For this review, take the finished solid that the model builds, in its own axes (mm). A direction names the side the tool comes from. Give positions to 0.01 mm unless a question says otherwise; leave off trailing zeros. Order: outer loops, then holes, each group sorted by start corner. A loop starts at its lowest first (then second) coordinate and runs counter-clockwise, first axis right, second up.
Autodesk Inventor part; units mm, degrees
ref_plane "YZ Plane" through (0, 0, 0) normal (1, 0, 0) x (0, 1, 0)
ref_plane "XZ Plane" through (0, 0, 0) normal (0, 1, 0) x (-1, 0, 0)
ref_plane "XY Plane" through (0, 0, 0) normal (0, 0, 1) x (1, 0, 0)
sketch "Sketch1" plane through (0, 0, 0) normal (0, 0, 1) x (1, 0, 0)
  line L0 (-12.7, -25.4) -> (12.7, -25.4)
  line L1 (12.7, -25.4) -> (12.7, 25.4)
  line L2 (12.7, 25.4) -> (-12.7, 25.4)
  line L3 (-12.7, 25.4) -> (-12.7, -25.4)
  line L4 (-12.7, -25.4) -> (12.7, 25.4) construction
  line L5 (12.7, -25.4) -> (-12.7, 25.4) construction
  line L6 (-10.16, -22.86) -> (10.16, -22.86)
  line L7 (10.16, -22.86) -> (10.16, 22.86)
  line L8 (10.16, 22.86) -> (-10.16, 22.86)
  line L9 (-10.16, 22.86) -> (-10.16, -22.86)
  line L10 (-10.16, -22.86) -> (10.16, 22.86) construction
  line L11 (10.16, -22.86) -> (-10.16, 22.86) construction
  point P0 (0, 0)
  dimension "d0" = 25.4
  dimension "d1" = 50.8
  dimension "d2" = 20.32
  dimension "d3" = 45.72
extrude "Extrusion1" add sketch "Sketch1" along normal mid plane 101.6
sketch "Sketch2" plane through (-12.7, 25.4, 50.8) normal (0, 1, 0) x (1, 0, 0)
  line L0 (25.4, 101.6) -> (25.4, 0)
  line L1 (25.4, 0) -> (0, 0)
  point P0 (12.7, 50.8)
  point P1 (12.7, 12.7)
  dimension "d6" = 12.7
  dimension "d7" = 12.7
hole "Hole1" at (0, 25.4, 38.1) direction (0, -1, 0) diameter 4.1402 end through all
pattern_linear "Rectangular Pattern1" count 4 spacing 25.4 along (0, 0, -1) of "Hole1"
properties part number "Drivetrain_short_front"
1) We need section C-C on y = 17.5. Give the boundary of the cut face in (x, z).
Answer sheet:
outline: (-12.7, -50.8) - (-10.16, -50.8) - (-10.16, 50.8) - (-12.7, 50.8) - close; (10.16, -50.8) - (12.7, -50.8) - (12.7, 50.8) - (10.16, 50.8) - close
2) To check wall thickness, follow line 1 (Z direction, x = 0, y = 23.9); line 2 (X direction, y = -14, z = 21.5); line 3 (Y direction, x = 9.25, z = -41.5). State the ranges of each line that lie inside material, in increasing order.
Answer sheet:
line 1: z = -50.8 to -40.17, -36.03 to -14.77, -10.63 to 10.63, 14.77 to 36.03, 40.17 to 50.8
line 2: x = -12.7 to -10.16, 10.16 to 12.7
line 3: y = -25.4 to -22.86, 22.86 to 25.4
3) Clearance check with a flat-ended pin moving along its axis: pin 1 (3.5 mm diameter, centred on x = 0, z = 12.7, fed in from +Y). State where the tip first meets the part, or that it passes through.
Answer sheet:
pin 1: passes through
4) Draft analysis for pull direction Y (two halves, no side actions). For faces 3 (the face through (0, 25.4, -1)), 4 (the face through (0, 22.86, -1)), 5 (the face through (-10.16, 0, -1)), 6 (the face through (-1.399, 24.112, -14.226)), state which applies: +Y half, -Y half, draft (parallel to the pull), parting line (faces both ways), or undercut.
Answer sheet:
face 3: +Y half
face 4: undercut
face 5: undercut
face 6: draft
5) We need section A-A on x = 7. Give the boundary of the cut face in (y, z).
Answer sheet:
outline: (-25.4, -50.8) - (-22.86, -50.8) - (-22.86, 50.8) - (-25.4, 50.8) - close; (22.86, -50.8) - (25.4, -50.8) - (25.4, 50.8) - (22.86, 50.8) - close
6) We need section B-B on z = 12.7. Give the boundary of the cut face in (x, y), then the cut area to 3 significant figures.
Answer sheet:
outline: (-12.7, -25.4) - (-2.07, -25.4) - (-2.07, -22.86) - (-10.16, -22.86) - (-10.16, 22.86) - (-2.07, 22.86) - (-2.07, 25.4) - (-12.7, 25.4) - close; (2.07, -25.4) - (12.7, -25.4) - (12.7, 25.4) - (2.07, 25.4) - (2.07, 22.86) - (10.16, 22.86) - (10.16, -22.86) - (2.07, -22.86) - close
area: 340 mm2
7) We need section D-D on z = -44. Give the boundary of the cut face in (x, y).
Answer sheet:
outline: (-12.7, -25.4) - (12.7, -25.4) - (12.7, 25.4) - (-12.7, 25.4) - close; hole (-10.16, -22.86) - (10.16, -22.86) - (10.16, 22.86) - (-10.16, 22.86) - close
8) Tool access review of faces 1 (the face through (-0.09, -24.15, 10.63)), 2 (the face through (0, -22.86, -1)): name each direction out of +Z, -Z, +X, -X, +Y, -Y from which nothing blocks a thin tool from reaching the whole face with its end or side.
Answer sheet:
face 1: +Y, -Y
face 2: +Z, -Z
